from build123d import *

# Parameters (mm, degrees)
SKETCH_R        = 1.2
PAD_DEPTH       = 3
PAD001_DEPTH    = 10
FILLET_R        = 3
SKETCH002_R     = 2.5
POCKET_DEPTH    = 6
PAD002_DEPTH    = 7
SKETCH004_W     = 20
SKETCH004_H     = 4
POCKET001_DEPTH = 12
SKETCH006_R     = 1.2
POCKET002_DEPTH = 5


with BuildPart() as part:
    # Sketch → Pad (new body)
    with BuildSketch(Plane.XY):
        Polygon((0, 12), (0, 0), (-20, 0), (-20, 12), (-15, 19.412805), (-5, 19.412805), align=None)
        with Locations((-13, 4)):
            Circle(SKETCH_R, mode=Mode.SUBTRACT)
        with Locations((-7, 4)):
            Circle(SKETCH_R, mode=Mode.SUBTRACT)
    extrude(amount=PAD_DEPTH)

    # Sketch001 (on Face10 of Pad) → Pad001 (join)
    with BuildSketch(Plane.XY.offset(3)):
        Polygon((-14.90374, 19.331674), (-5.09626, 19.331674), (-1.5, 14), (-18.5, 14), align=None)
    extrude(amount=PAD001_DEPTH)

    # Fillet
    fillet_edges = [part.edges().sort_by_distance(p)[0] for p in [
        (-3.29813, 16.665837, 13),
        (-10, 19.331674, 13),
        (-16.70187, 16.665837, 13),
    ]]
    fillet(fillet_edges, radius=FILLET_R)

    # Sketch002 (on Face12 of Pad001) → Pocket (cut)
    with BuildSketch(Plane.XZ.offset(-14)):
        with Locations((-10, 8)):
            Circle(SKETCH002_R)
    extrude(amount=-POCKET_DEPTH, mode=Mode.SUBTRACT)

    # Sketch003 (on Face19 of Pocket) → Pad002 (join)
    with BuildSketch(Plane(origin=(0, 0, 0), x_dir=(1, 0, 0), z_dir=(0, 0, -1))):
        Polygon((0, 0), (-20, 0), (-20, -12), (-15.004024, -19.406839), (-4.995976, -19.406839), (0, -12), align=None)
    extrude(amount=PAD002_DEPTH)

    # Sketch004 (on Face22 of Pad002) → Pocket001 (cut)
    with BuildSketch(Plane.XZ):
        with Locations((-10, -2)):
            Rectangle(SKETCH004_W, SKETCH004_H)
    extrude(amount=-POCKET001_DEPTH, mode=Mode.SUBTRACT)

    # Sketch006 (on Face26 of Pocket001) → Pocket002 (cut)
    with BuildSketch(Plane(origin=(0, 0, -7), x_dir=(1, 0, 0), z_dir=(0, 0, -1))):
        with Locations((-13, -4)):
            Circle(SKETCH006_R)
        with Locations((-7, -4)):
            Circle(SKETCH006_R)
    extrude(amount=-POCKET002_DEPTH, mode=Mode.SUBTRACT)


solid = part.part
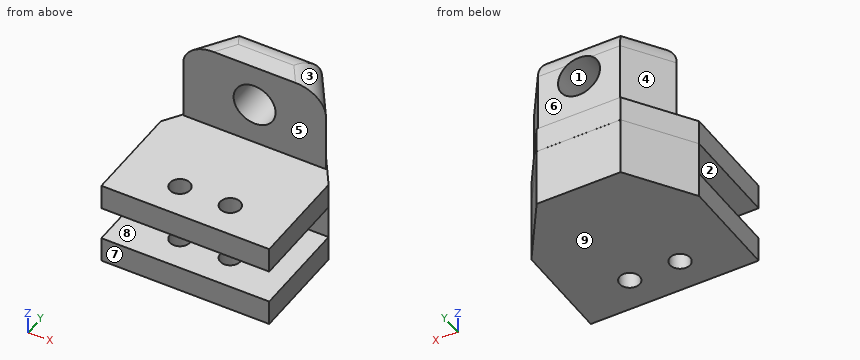
The model under review builds one solid part; all positions refer to its coordinate system, in mm. Face numbers are marked on the shaded views. A direction names the side the tool comes from. Round coordinates to 2 decimals unless told otherwise and drop trailing zeros. Loops run counter-clockwise (first coordinate to the right, second up) from the corner with the lowest first, then second, coordinate; pieces in that order, holes last. Notation, with made-up numbers: (-6.75, -34.5) -> (40.25, -34.5) arc R34 cw to (40.25, -3.5) -> close; hole circle Ø2 at (78, 14). An arc over 180 degrees is marked (long way). Write item = value, one per line. Start each with the question number.
Item 1: Take a section at C-C on y = 4. Give the boundary of the cut face in (x, z), plus the area to 3 significant figures.
Item 2: Take a section at B-B on x = -7. Count the separate pieces of the cut face and the enclosed holes in it, plus the area to 3 significant figures.
Item 3: To check wall thickness, follow L1, parallel to Z at x = -15.5, y = 5.5; L2, parallel to X at y = 4, z = -5.75; L3, parallel to Y at x = -7, z = -6. State the ranges of each line that lie inside material, in increasing order.
Item 4: Mouldability with a two-part tool opening along X and no side actions: class the marked faces 1, 2, 3 and 4 as released by +X, released by -X, zero draft, split by the parting line, or undercut.
Item 5: For the marked faces 5, 6, 7, 8 and 9, list the 3-axis set-ups (+Z, -Z, +X, -X, +Y, -Y) from which the entire face can be reached by the end or side of a thin tool; tool diameter is ignored.
Item 6: Insertion check: pin 1 (1.5 mm diameter, centred on x = -9, z = 5.5, fed in from +Y); pin 2 (3 mm diameter, centred on x = -7, y = 4, fed in from +Z); pin 3 (6 mm diameter, centred on x = -10, z = 8, fed in from -Y). Each pin has a flat end and moves straight along its axis. Give the tip position at first contact, or say it passes through.
Item 7: Take a section at A-A on y = 10.5. Give the boundary of the cut face in (x, z), plus the area to 3 significant figures.
Result:
q1.outline = (-20, -7) -> (-14.2, -7) -> (-14.2, -4) -> (-20, -4) -> close; (-20, 0) -> (-14.2, 0) -> (-14.2, 3) -> (-20, 3) -> close; (-11.8, -7) -> (-8.2, -7) -> (-8.2, -4) -> (-11.8, -4) -> close; (-11.8, 0) -> (-8.2, 0) -> (-8.2, 3) -> (-11.8, 3) -> close; (-5.8, -7) -> (0, -7) -> (0, -4) -> (-5.8, -4) -> close; (-5.8, 0) -> (0, 0) -> (0, 3) -> (-5.8, 3) -> close
q1.area = 91.2 mm²
q2.separate_pieces = 3
q2.enclosed_holes = 0
q2.area = 183 mm²
q3.L1 = -7 to -4, 0 to 3
q3.L2 = -20 to -14.2, -11.8 to -8.2, -5.8 to 0
q3.L3 = 0 to 2.8, 5.2 to 19.41
q4.face_1 = undercut
q4.face_2 = zero draft
q4.face_3 = released by +X
q4.face_4 = released by -X
q5.face_5 = +Z, +X, -X, -Y
q5.face_6 = +Z, +X, -X, +Y
q5.face_7 = +Z, -Z, +X, -X, -Y
q5.face_8 = +X, -X, -Y
q5.face_9 = -Z, +X, -X, +Y, -Y
q6.pin_1 = 19.33
q6.pin_2 = 3
q6.pin_3 = 14
q7.outline = (-20, -7) -> (0, -7) -> (0, -4) -> (-20, -4) -> close; (-20, 0) -> (0, 0) -> (0, 3) -> (-20, 3) -> close
q7.area = 120 mm²
